Check sheet for the modelled part. Datum: model origin and axes. Units: mm. Round coordinates to 2 decimals unless told otherwise and drop trailing zeros. Order: outer loops, then holes, each group sorted by start corner. A loop starts at its lowest first (then second) coordinate and runs counter-clockwise, first axis right, second up. Notation, with made-up numbers: (-2, -24.75) -> (53, -24.75) arc R27 cw to (53, -7.75) -> close; hole circle Ø3 at (-38.5, 20). An arc over 180 degrees is marked (long way). Answer as CSV lines item,"result". Start each with the question number.
from build123d import *

# Parameters (mm, degrees)
F0_W     = 50
F0_H     = 14
F0_R     = 1.65
F0_R_2   = 1.7
F0_R_3   = 1.75
F0_R_4   = 1.8
F0_R_5   = 1.85
F0_R_6   = 1.9
F0_R_7   = 1.95
F0_R_8   = 2
F0_R_9   = 1.25
F0_R_10  = 1.3
F0_R_11  = 1.35
F0_R_12  = 1.4
F0_R_13  = 1.45
F0_R_14  = 1.5
F0_R_15  = 1.55
F0_R_16  = 1.6
F1_DEPTH = 5


with BuildPart() as f1:
    # F0 (on Top) → F1 (new body)
    with BuildSketch(Plane.XY):
        Rectangle(F0_W, F0_H)
        with Locations((-21, -3)):
            Circle(F0_R, mode=Mode.SUBTRACT)
        with Locations((-15, -3)):
            Circle(F0_R_2, mode=Mode.SUBTRACT)
        with Locations((-9, -3)):
            Circle(F0_R_3, mode=Mode.SUBTRACT)
        with Locations((-3, -3)):
            Circle(F0_R_4, mode=Mode.SUBTRACT)
        with Locations((3, -3)):
            Circle(F0_R_5, mode=Mode.SUBTRACT)
        with Locations((9, -3)):
            Circle(F0_R_6, mode=Mode.SUBTRACT)
        with Locations((15, -3)):
            Circle(F0_R_7, mode=Mode.SUBTRACT)
        with Locations((21, -3)):
            Circle(F0_R_8, mode=Mode.SUBTRACT)
        with Locations((-21, 3)):
            Circle(F0_R_9, mode=Mode.SUBTRACT)
        with Locations((-15, 3)):
            Circle(F0_R_10, mode=Mode.SUBTRACT)
        with Locations((-9, 3)):
            Circle(F0_R_11, mode=Mode.SUBTRACT)
        with Locations((-3, 3)):
            Circle(F0_R_12, mode=Mode.SUBTRACT)
        with Locations((3, 3)):
            Circle(F0_R_13, mode=Mode.SUBTRACT)
        with Locations((9, 3)):
            Circle(F0_R_14, mode=Mode.SUBTRACT)
        with Locations((15, 3)):
            Circle(F0_R_15, mode=Mode.SUBTRACT)
        with Locations((21, 3)):
            Circle(F0_R_16, mode=Mode.SUBTRACT)
    extrude(amount=-F1_DEPTH)


solid = f1.part
1) Material ranges on line 1 along Y through (x, z) = (-15, -3.85); line 2 along Y through (x, z) = (3, -4.8); line 3 along Y through (x, z) = (-7.5, -3.65), recorded low to high.
2) Section check D-D on x = 9. Record the cut outline in (y, z), then the cut area to 3 significant figures.
3) Section check A-A on x = -15. Record the cut outline in (y, z).
4) Section check B-B on z = -1.6. Count the separate pieces of the cut face and the enclosed holes in it, then the cut area to 3 significant figures.
5) Mould release check, pull along X, two halves, no side actions. Record for faces 1 (the face through (-7.753, 2.483, -2.465)), 2 (the face through (25, 0, -2)), 3 (the face through (-25, 0, -2)), 4 (the face through (-13.38, -2.49, -2.46)): released by +X, released by -X, zero draft, split by the parting line, or undercut.
Solutions:
1,line 1,"y = -7 to -4.7, -1.3 to 1.7, 4.3 to 7"
1,line 2,"y = -7 to -4.85, -1.15 to 1.55, 4.45 to 7"
1,line 3,"y = -7 to -3.9, -2.1 to 7"
2,outline,"(-7, -5) -> (-4.9, -5) -> (-4.9, 0) -> (-7, 0) -> close; (-1.1, -5) -> (1.5, -5) -> (1.5, 0) -> (-1.1, 0) -> close; (4.5, -5) -> (7, -5) -> (7, 0) -> (4.5, 0) -> close"
2,area,"36.0 mm^2"
3,outline,"(-7, -5) -> (-4.7, -5) -> (-4.7, 0) -> (-7, 0) -> close; (-1.3, -5) -> (1.7, -5) -> (1.7, 0) -> (-1.3, 0) -> close; (4.3, -5) -> (7, -5) -> (7, 0) -> (4.3, 0) -> close"
4,separate pieces,"1"
4,enclosed holes,"16"
4,area,"565 mm^2"
5,face 1,"undercut"
5,face 2,"released by +X"
5,face 3,"released by -X"
5,face 4,"undercut"
